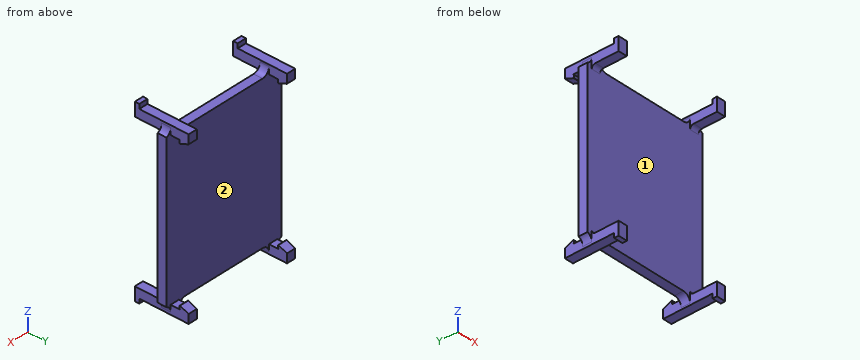
from build123d import *

# Parameters (mm, degrees)
SKETCH1_W           = 44.45
SKETCH1_H           = 53.594
BOSS_EXTRUDE1_DEPTH = 3.175
SKETCH2_W           = 3.175
SKETCH2_H           = 19.05
BOSS_EXTRUDE2_DEPTH = 3.175
SKETCH4_W           = 3.175
SKETCH4_H           = 19.05
BOSS_EXTRUDE3_DEPTH = 3.175
BOSS_EXTRUDE4_DEPTH = 3.175
BOSS_EXTRUDE5_DEPTH = 3.175
SKETCH11_W          = 3.175
SKETCH11_H          = 1.5875
BOSS_EXTRUDE6_DEPTH = 1.5875
SKETCH12_W          = 3.175
SKETCH12_H          = 1.5875
BOSS_EXTRUDE7_DEPTH = 1.5875
FILLET1_R           = 2.54
FILLET2_R           = 0.127
FILLET3_R           = 1.27


with BuildPart() as part:
    # Sketch1 → Boss-Extrude1 (new body)
    with BuildSketch(Plane(origin=(0, 0, 0), x_dir=(1, 0, 0), z_dir=(0, 1, 0))):
        with Locations((20.14322973, 10.682587838)):
            Rectangle(SKETCH1_W, SKETCH1_H)
    extrude(amount=BOSS_EXTRUDE1_DEPTH)

    # Sketch2 → Boss-Extrude2 (add)
    with BuildSketch(Plane.XY.offset(16.114412162)):
        with Locations((1.09322973, 0)):
            Rectangle(SKETCH2_W, SKETCH2_H)
        with Locations((39.19322973, 0)):
            Rectangle(SKETCH2_W, SKETCH2_H)
    extrude(amount=BOSS_EXTRUDE2_DEPTH)

    # Sketch4 → Boss-Extrude3 (add)
    with BuildSketch(Plane(origin=(0, 0, -37.479587838), x_dir=(-1, 0, 0), z_dir=(0, 0, -1))):
        with Locations((-1.09322973, 0)):
            Rectangle(SKETCH4_W, SKETCH4_H)
        with Locations((-39.19322973, 0)):
            Rectangle(SKETCH4_W, SKETCH4_H)
    extrude(amount=BOSS_EXTRUDE3_DEPTH)

    # Sketch9 → Boss-Extrude4 (add)
    with BuildSketch(Plane(origin=(40.78072973, 0, 0), x_dir=(0, 0, -1), z_dir=(1, 0, 0))):
        with BuildLine():
            Line((-16.114412162, 9.525), (-14.844412162, 6.35))
            add(Edge.make_bspline(
                [(-14.844412162, 6.35), (-15.980974803, 6.259875381), (-16.114412162, 6.477)],
                knots=[0, 0, 0, 1, 1, 1], degree=2))
            Line((-16.114412162, 6.477), (-16.114412162, 9.525))
        make_face()
        with BuildLine():
            Line((37.479587838, 9.525), (36.209587838, 6.35))
            add(Edge.make_bspline(
                [(36.209587838, 6.35), (37.346150478, 6.259875381), (37.479587838, 6.477)],
                knots=[0, 0, 0, 1, 1, 1], degree=2))
            Line((37.479587838, 6.477), (37.479587838, 9.525))
        make_face()
    extrude(amount=-BOSS_EXTRUDE4_DEPTH)

    # Sketch10 → Boss-Extrude5 (add)
    with BuildSketch(Plane.ZY.offset(0.49427027)):
        with BuildLine():
            Line((-37.479587838, 9.525), (-36.209587838, 6.35))
            add(Edge.make_bspline(
                [(-36.209587838, 6.35), (-37.253478126, 6.221904512), (-37.479587838, 6.477)],
                knots=[0, 0, 0, 1, 1, 1], degree=2))
            Line((-37.479587838, 6.477), (-37.479587838, 9.525))
        make_face()
        with BuildLine():
            Line((16.114412162, 9.525), (14.844412162, 6.35))
            add(Edge.make_bspline(
                [(14.844412162, 6.35), (15.88830245, 6.221904512), (16.114412162, 6.477)],
                knots=[0, 0, 0, 1, 1, 1], degree=2))
            Line((16.114412162, 6.477), (16.114412162, 9.525))
        make_face()
    extrude(amount=-BOSS_EXTRUDE5_DEPTH)

    # Sketch11 → Boss-Extrude6 (add)
    with BuildSketch(Plane.XY.offset(19.289412162)):
        with Locations((1.09322973, -8.73125)):
            Rectangle(SKETCH11_W, SKETCH11_H)
        with Locations((39.19322973, -8.73125)):
            Rectangle(SKETCH11_W, SKETCH11_H)
    extrude(amount=BOSS_EXTRUDE6_DEPTH)

    # Sketch12 → Boss-Extrude7 (add)
    with BuildSketch(Plane(origin=(0, 0, -40.654587838), x_dir=(-1, 0, 0), z_dir=(0, 0, -1))):
        with Locations((-39.19322973, -8.73125)):
            Rectangle(SKETCH12_W, SKETCH12_H)
        with Locations((-1.09322973, -8.73125)):
            Rectangle(SKETCH12_W, SKETCH12_H)
    extrude(amount=BOSS_EXTRUDE7_DEPTH)

    # Fillet1
    # the kernel refuses this fillet: 2.54 mm, written as the material it adds along each edge
    with BuildSketch(Plane(origin=(37.60572973, 0, 16.114412162), x_dir=(0, 0, 1), z_dir=(0, 1, 0)), Plane(origin=(2.68072973, 0, -37.479587838), x_dir=(0, 0, -1), z_dir=(0, 1, 0))) as fillet1_piece_1:
        with BuildLine():
            CenterArc((FILLET1_R, -FILLET1_R), FILLET1_R, 90, 90)
            Line((0, -FILLET1_R), (0, 0))
            Line((0, 0), (FILLET1_R, 0))
        make_face()
    extrude(amount=3.175)
    with BuildSketch(Plane(origin=(40.78072973, 3.175, 16.114412162), x_dir=(1, 0, 0), z_dir=(0, -1, 0)), Plane(origin=(-0.49427027, 0, 16.114412162), x_dir=(-1, 0, 0), z_dir=(0, 1, 0)), Plane(origin=(-0.49427027, 3.175, -37.479587838), x_dir=(-1, 0, 0), z_dir=(0, -1, 0))) as fillet1_piece_2:
        with BuildLine():
            CenterArc((2.54, 2.35464302), FILLET1_R, 180, 67.975687163)
            Line((0, 2.35464302), (0, 0))
            Line((0, 0), (1.5875, 0))
        make_face()
    extrude(amount=3.175)
    with BuildSketch(Plane(origin=(2.68072973, 3.175, 16.114412162), x_dir=(1, 0, 0), z_dir=(0, -1, 0)), Plane(origin=(37.60572973, 3.175, -37.479587838), x_dir=(-1, 0, 0), z_dir=(0, -1, 0))) as fillet1_piece_3:
        with BuildLine():
            CenterArc((FILLET1_R, FILLET1_R), FILLET1_R, 180, 90)
            Line((0, FILLET1_R), (0, 0))
            Line((0, 0), (FILLET1_R, 0))
        make_face()
    extrude(amount=3.175)
    with BuildSketch(Plane(origin=(40.78072973, 0, -37.479587838), x_dir=(0, 0, -1), z_dir=(0, 1, 0))) as fillet1_piece_4:
        with BuildLine():
            CenterArc((2.35464302, -2.54), FILLET1_R, 90, 67.975687163)
            Line((0, -1.5875), (0, 0))
            Line((0, 0), (2.35464302, 0))
        make_face()
    extrude(amount=3.175)

    # Fillet2
    fillet2_edges = [part.edges().sort_by_distance(p)[0] for p in [
        (39.19322973, 6.35, 14.844412162),
        (39.19322973, 6.35, -36.209587838),
        (1.09322973, 6.35, -36.209587838),
        (1.09322973, 6.35, 14.844412162),
    ]]
    fillet(fillet2_edges, radius=FILLET2_R)

    # Fillet3
    fillet3_edges = [part.edges().sort_by_distance(p)[0] for p in [
        (1.09322973, 0, 16.114412162),
        (39.19322973, 0, 16.114412162),
        (39.19322973, 0, -37.479587838),
        (1.09322973, 0, -37.479587838),
    ]]
    fillet(fillet3_edges, radius=FILLET3_R)


solid = part.part
The listing builds one solid part. Answer for the finished solid, in the listing's coordinates (mm). Face numbers are marked on the shaded views. Give positions to 0.01 mm unless a question says otherwise; leave off trailing zeros. Write each loop counter-clockwise with the first axis right and the second up, starting at its lowest first coordinate (ties: lowest second). Pieces come first, ordered by that corner, then holes.
1) Section D-D (x = 20) is taken. Write down the section's boundary in (y, z) (3 decimals).
2) Given P1, Ø12, axis at x = 36, z = -28.5, coming from the -Y side; P2, Ø2.5, axis at x = 0.5, y = -3.5, coming from the +Z side; P3, Ø1.6, axis at x = 1.5, y = 3.5, coming from the -Z side, each flat-ended and moving along its own axis, determine where each tip first touches the part or whether it passes through.
3) Section B-B (y = 2.5) is taken. Write down the section's boundary in (x, z).
4) Find the intervals of material crossed by L1, parallel to Z at x = 38.5, y = -8.25; L2, parallel to Z at x = 2, y = -5.25; L3, parallel to Y at x = 32, z = 2 (3 decimals), in increasing order.
5) Section C-C (z = -7) is taken. Write down the section's boundary in (x, y) (3 decimals).
6) Section A-A (y = -5.25) is taken. Write down the section's boundary in (x, z).
7) For a pull along Z with two mould halves and no side action, classify the marked faces 1 and 2 as pulls with the +Z half, pulls with the -Z half, needs draft (parallel to the pull), parting line crosses it, or undercut.
Response:
1. outline: (0, -37.48) - (3.175, -37.48) - (3.175, 16.114) - (0, 16.114) - close
2. P1: stops at y = 0
2. P2: stops at z = 19.29
2. P3: stops at z = -40.65
3. outline: (-2.08, -37.48) arc R2.54 cw to (-0.49, -39.83) - (-0.49, -40.65) - (2.68, -40.65) - (2.68, -40.02) arc R2.54 cw to (5.22, -37.48) - (35.07, -37.48) arc R2.54 cw to (37.61, -40.02) - (37.61, -40.65) - (40.78, -40.65) - (40.78, -39.83) arc R2.54 cw to (42.37, -37.48) - (42.37, 16.11) arc R2.54 cw to (40.78, 18.47) - (40.78, 19.29) - (37.61, 19.29) - (37.61, 18.65) arc R2.54 cw to (35.07, 16.11) - (5.22, 16.11) arc R2.54 cw to (2.68, 18.65) - (2.68, 19.29) - (-0.49, 19.29) - (-0.49, 18.47) arc R2.54 cw to (-2.08, 16.11) - close
4. L1: z = -42.24 to -37.48, 16.11 to 20.88
4. L2: z = -40.65 to -37.48, 16.11 to 19.29
4. L3: y = 0 to 3.175
5. outline: (-2.082, 0) - (42.368, 0) - (42.368, 3.175) - (-2.082, 3.175) - close
6. outline: (-0.49, -40.65) - (2.68, -40.65) - (2.68, -37.48) - (-0.49, -37.48) - close; (-0.49, 16.11) - (2.68, 16.11) - (2.68, 19.29) - (-0.49, 19.29) - close; (37.61, -40.65) - (40.78, -40.65) - (40.78, -37.48) - (37.61, -37.48) - close; (37.61, 16.11) - (40.78, 16.11) - (40.78, 19.29) - (37.61, 19.29) - close
7. face 1: undercut
7. face 2: undercut
